Geometry check sheet. Reference: drawing and pictorial views, mm from the part's lowest x, y, z. Give positions to 0.01 mm unless a question says otherwise; leave off trailing zeros. Loops run counter-clockwise (first coordinate to the right, second up) from the corner with the lowest first, then second, coordinate; pieces in that order, holes last. Notation, with made-up numbers: (-6.5, -36.5) -> (29.5, -36.5) arc R17 ccw to (29.5, -5.5) -> close; hole circle Ø8 at (7, 32). An arc over 180 degrees is marked (long way). One line per item, written item: value. Start each with the question number.
(1) Draft check along Y on the marked faces 1, 2 and 3. Enter one of: pulls with the +Y half, pulls with the -Y half, needs draft (parallel to the pull), parting line crosses it, or undercut.
(2) Scan lines: line 1 along Y through (x, z) = (3.5, 0.7); line 2 along X through (y, z) = (2.1, 0.15); line 3 along X through (y, z) = (3.7, 0.3). Record each from-to range of solid material in increasing order. Write a range as from..to.
(3) Sectioned sample at B-B, the plane y = 3. Record the cut outline in (x, z).
(4) Sectioned sample at A-A, the plane x = 3.5. Record the cut outline in (y, z), then the cut area to 3 significant figures.
(5) Sectioned sample at C-C, the plane z = 0.15. Record the cut outline in (x, y).
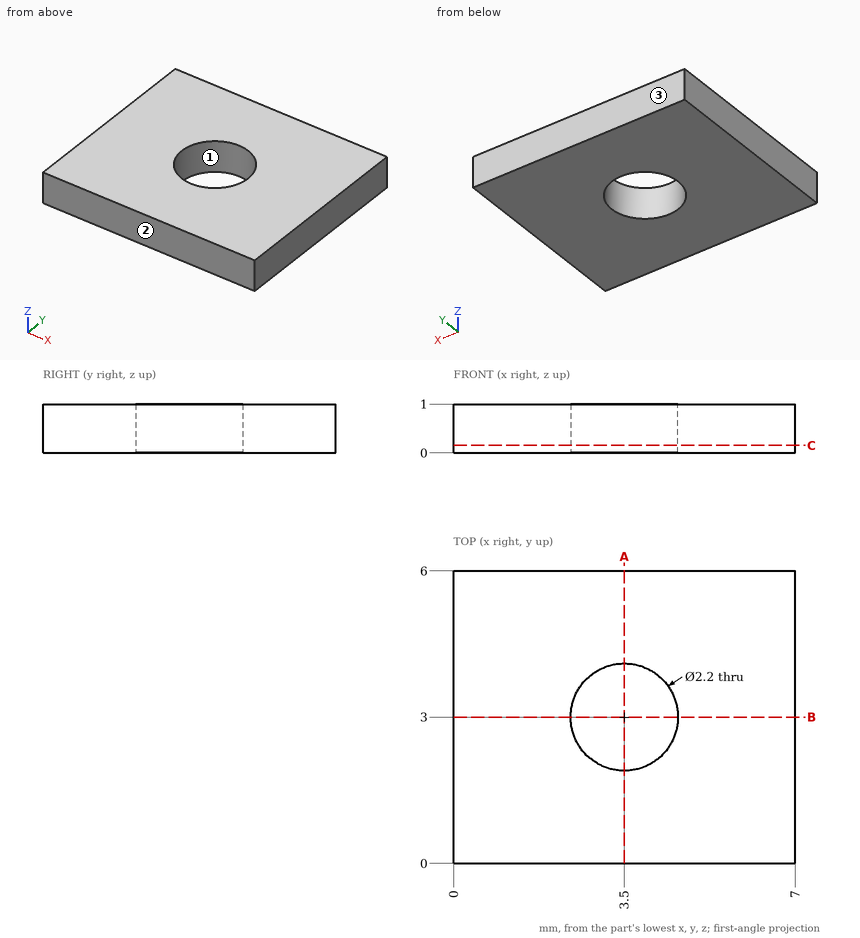
Calculated:
1. face 1: undercut
1. face 2: pulls with the -Y half
1. face 3: pulls with the +Y half
2. line 1: y = 0..1.9, 4.1..6
2. line 2: x = 0..2.87, 4.13..7
2. line 3: x = 0..2.65, 4.35..7
3. outline: (0, 0) -> (2.4, 0) -> (2.4, 1) -> (0, 1) -> close; (4.6, 0) -> (7, 0) -> (7, 1) -> (4.6, 1) -> close
4. outline: (0, 0) -> (1.9, 0) -> (1.9, 1) -> (0, 1) -> close; (4.1, 0) -> (6, 0) -> (6, 1) -> (4.1, 1) -> close
4. area: 3.80 mm2
5. outline: (0, 0) -> (7, 0) -> (7, 6) -> (0, 6) -> close; hole circle Ø2.2 at (3.5, 3)
